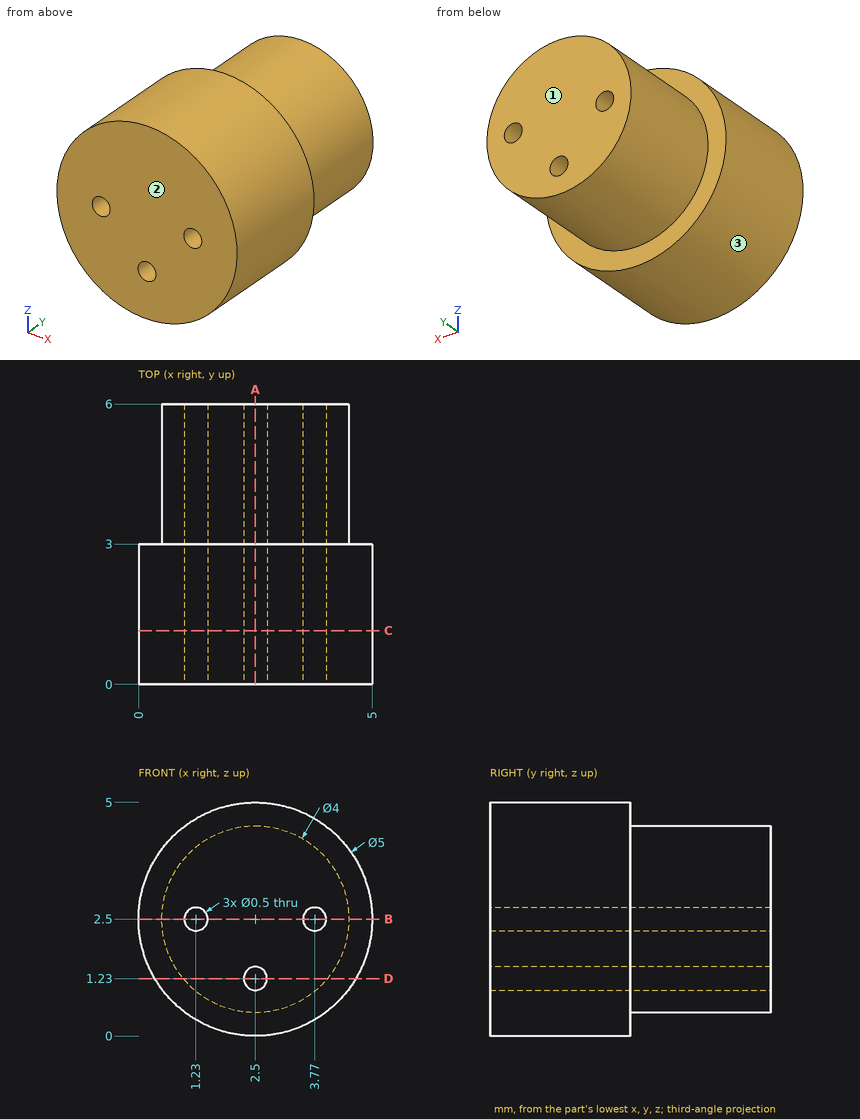
The figure shows three views and two pictorial views of one solid part (mm, origin at its lowest corner). Answer the questions. Give positions to 0.01 mm unless a question says otherwise; leave off trailing zeros. Order: outer loops, then holes, each group sorted by start corner. A loop starts at its lowest first (then second) coordinate and runs counter-clockwise, first axis right, second up. Notation, with made-up numbers: (48, 14.25) -> (85, 14.25) arc R29 ccw to (85, 43.25) -> close; hole circle Ø8 at (64, 43). An arc over 180 degrees is marked (long way). Answer as CSV lines item,"result". Start each with the question number.
Q1. Determine the mould class of the marked faces 1, 2 and 3 for opening direction Y: pulls with the +Y half, pulls with the -Y half, needs draft (parallel to the pull), parting line crosses it, or undercut.
Q2. A cutting plane is placed at A-A (x = 2.5). Determine the outline of the cut face in (y, z).
Q3. A cutting plane is placed at C-C (y = 1.15). Determine the outline of the cut face in (x, z).
Q4. A cutting plane is placed at B-B (z = 2.5). Determine the outline of the cut face in (x, y).
Q5. Find the intervals of material crossed by L1, parallel to X at y = 2.95, z = 2.5; L2, parallel to X at y = 4.45, z = 2.5; L3, parallel to Y at x = 0.6, z = 3.75, in increasing order.
Q6. A cutting plane is placed at D-D (z = 1.23). Determine the outline of the cut face in (x, y).
Results found:
1,face 1,"pulls with the +Y half"
1,face 2,"pulls with the -Y half"
1,face 3,"needs draft"
2,outline,"(0, 0) -> (3, 0) -> (3, 0.5) -> (6, 0.5) -> (6, 0.98) -> (0, 0.98) -> close; (0, 1.48) -> (6, 1.48) -> (6, 4.5) -> (3, 4.5) -> (3, 5) -> (0, 5) -> close"
3,outline,"circle Ø5 at (2.5, 2.5); hole circle Ø0.5 at (1.23, 2.5); hole circle Ø0.5 at (2.5, 1.23); hole circle Ø0.5 at (3.77, 2.5)"
4,outline,"(0, 0) -> (0.98, 0) -> (0.98, 6) -> (0.5, 6) -> (0.5, 3) -> (0, 3) -> close; (1.48, 0) -> (3.52, 0) -> (3.52, 6) -> (1.48, 6) -> close; (4.02, 0) -> (5, 0) -> (5, 3) -> (4.5, 3) -> (4.5, 6) -> (4.02, 6) -> close"
5,L1,"0 to 0.98, 1.48 to 3.52, 4.02 to 5"
5,L2,"0.5 to 0.98, 1.48 to 3.52, 4.02 to 4.5"
5,L3,"0 to 3"
6,outline,"(0.35, 0) -> (2.25, 0) -> (2.25, 6) -> (0.95, 6) -> (0.95, 3) -> (0.35, 3) -> close; (2.75, 0) -> (4.65, 0) -> (4.65, 3) -> (4.05, 3) -> (4.05, 6) -> (2.75, 6) -> close"
